Geometry check sheet. Reference: the model listing, model coordinates, mm. A direction names the side the tool comes from. Coordinates: 2 decimals unless noted, no trailing zeros. Order: outer loops, then holes, each group sorted by start corner. A loop starts at its lowest first (then second) coordinate and runs counter-clockwise, first axis right, second up. Notation, with made-up numbers: (16.25, 0.5) - (32.25, 0.5) arc R11 cw to (32.25, 12.5) - close; hole circle Ø6 at (-20, 3). An arc over 180 degrees is marked (long way). Return JSON: item names as keys, results as strings. Group by question number.
Item 1: Section check C-C on z = 161.5. Enter the section's corners in (x, y) (3 decimals), then the cut area to 3 significant figures.
Item 2: Draft check along Y on faces 1 (the flat face through (0, -554.51, 310)), 2 (the flat face through (0, 3.155, 163)), 3 (the flat face through (0, -548.2, 303)), 4 (the flat face through (-25.4, -341, 325)). Enter one of: pulls with the +Y half, pulls with the -Y half, needs draft (parallel to the pull), parting line crosses it, or undercut.
Item 3: Section check A-A on z = 47.5. Enter the section's corners in (x, y) (3 decimals).
Item 4: Gauge pin test, flat ends, axial feed: pin 1 (16 mm diameter, centred on x = 0, y = -600.505, fed in from +Z); pin 2 (2 mm diameter, centred on x = 17.5, y = -489, fed in from -Z); pin 3 (15 mm diameter, centred on x = -8, z = 236, fed in from -Y) (3 decimals). Record the tip position at first contact, or that the pin passes through.
Item 5: Tool access check on faces 5 (the flat face through (0, -592, 282.58)), 6 (the flat face through (0, -595, 288.89)), 7 (the flat face through (0, -279, 324.39)). Record the directions out of +Z, -Z, +X, -X, +Y, -Y that give a thin tool (end or side, any length) a straight path to the whole face; none if there is none.
Item 6: Section check B-B on y = -520.5. Enter the section's corners in (x, z).
Item 7: Scan lines: probe 1 along Y at (x, z) = (0, 285.75) (3 decimals); probe 2 along X at (y, z) = (1.25, 47.5); probe 3 along Y at (x, z) = (19, 296) (3 decimals). Record each from-to range of solid material in increasing order.
from build123d import *

# Parameters (mm, degrees)
CROQUIS1_W              = 50.8
CROQUIS1_H              = 6.31
SALIENTE_EXTRUIR1_DEPTH = 330.7
CROQUIS3_W              = 50.8
CROQUIS3_H              = 6.31
SALIENTE_EXTRUIR2_DEPTH = 538.2
CROQUIS7_W              = 50.8
CROQUIS7_H              = 6.31
CROQUIS8_R              = 5
CORTAR_EXTRUIR2_DEPTH   = 15.875
CROQUIS9_R              = 6.5
CORTAR_EXTRUIR3_DEPTH   = 15.875
CROQUIS11_R             = 5
CORTAR_EXTRUIR5_DEPTH   = 10


with BuildPart() as part:
    # Croquis1 → Saliente-Extruir1 (new body)
    with BuildSketch(Plane.XY):
        Rectangle(CROQUIS1_W, CROQUIS1_H)
    extrude(amount=SALIENTE_EXTRUIR1_DEPTH)

    # Croquis3 → Saliente-Extruir2 (add)
    with BuildSketch(Plane.XZ.offset(3.155)):
        with Locations((0, 327.545)):
            Rectangle(CROQUIS3_W, CROQUIS3_H)
    extrude(amount=SALIENTE_EXTRUIR2_DEPTH)

    # Barrer1: sweep along a curve in space
    with BuildLine() as barrer1_path:
        Line((0, -541.355, 327.545), (0, -551.355, 327.545))
        Line((0, -551.355, 327.545), (0, -551.355, 285.735))
        Line((0, -551.355, 285.735), (0, -634.515, 285.735))
    # Croquis7 → Barrer1 (sweep)
    with BuildSketch(Plane.XZ.offset(541.355)):
        with Locations((0, 327.545)):
            Rectangle(CROQUIS7_W, CROQUIS7_H)
    sweep(path=barrer1_path.line, transition=Transition.RIGHT)

    # Croquis8 → Cortar-Extruir2 (cut)
    with BuildSketch(Plane(origin=(0, 0, 282.58), x_dir=(-1, 0, 0), z_dir=(0, 0, -1))):
        with Locations((0, -600.505)):
            Circle(CROQUIS8_R)
    extrude(amount=-CORTAR_EXTRUIR2_DEPTH, mode=Mode.SUBTRACT)

    # Croquis9 → Cortar-Extruir3 (cut)
    with BuildSketch(Plane(origin=(0, 3.155, 0), x_dir=(1, 0, 0), z_dir=(0, 1, 0))):
        with Locations(Location((0, -47.5, 0), (0, 0, 270))):
            Circle(CROQUIS9_R)
        with Locations(Location((0, -16.5, 0), (0, 0, 270))):
            Circle(CROQUIS9_R)
    extrude(amount=-CORTAR_EXTRUIR3_DEPTH, mode=Mode.SUBTRACT)

    # Croquis11 → Cortar-Extruir5 (cut)
    with BuildSketch(Plane(origin=(0, 3.155, 0), x_dir=(1, 0, 0), z_dir=(0, 1, 0))):
        with Locations(Location((0, -244.19, 0), (0, 0, 270))):
            Circle(CROQUIS11_R)
    extrude(amount=-CORTAR_EXTRUIR5_DEPTH, mode=Mode.SUBTRACT)


solid = part.part
Computed:
{
 "1": {"outline": "(-25.4, -3.155) - (25.4, -3.155) - (25.4, 3.155) - (-25.4, 3.155) - close", "area": "321 mm²"},
 "2": {"face 1": "pulls with the -Y half", "face 2": "pulls with the +Y half", "face 3": "undercut", "face 4": "needs draft"},
 "3": {"outline": "(-25.4, -3.155) - (-6.5, -3.155) - (-6.5, 3.155) - (-25.4, 3.155) - close; (6.5, -3.155) - (25.4, -3.155) - (25.4, 3.155) - (6.5, 3.155) - close"},
 "4": {"pin 1": "stops at z = 288.89", "pin 2": "stops at z = 324.39", "pin 3": "stops at y = -3.155"},
 "5": {"face 5": "-Z, +X, -X, -Y", "face 6": "+Z, +X, -X, -Y", "face 7": "-Z, +X, -X"},
 "6": {"outline": "(-25.4, 324.39) - (25.4, 324.39) - (25.4, 330.7) - (-25.4, 330.7) - close"},
 "7": {"probe 1": "y = -634.515 to -605.505, -595.505 to -548.2, -3.155 to 3.155", "probe 2": "x = -25.4 to -6.5, 6.5 to 25.4", "probe 3": "y = -554.51 to -548.2, -3.155 to 3.155"}
}
